Work out the finished part from the listing and answer in its coordinate system (mm). A direction names the side the tool comes from. Coordinates: 2 decimals unless noted, no trailing zeros. Order: outer loops, then holes, each group sorted by start corner. A loop starts at its lowest first (then second) coordinate and runs counter-clockwise, first axis right, second up. Notation, with made-up numbers: (0, 69) -> (55, 69) arc R17 ccw to (55, 75) -> close; hole circle Ø8 at (7, 47.25). An arc over 180 degrees is marked (long way). Answer as CSV lines item,"result". Start each with the question number.
Item 1: Section A-A (y = -0.5) is taken. Write down the section's boundary in (x, z), then the cut area to 3 significant figures.
Item 2: For a pull along X with two mould halves and no side action, classify faces 3 (the face through (3, 4.226, -5)), 4 (the face through (25.591, -5, -5)), 5 (the face through (-22.034, -5, -5)), 6 (the face through (3, 5, -381)) as pulls with the +X half, pulls with the -X half, needs draft (parallel to the pull), parting line crosses it, or undercut.
Item 3: Section B-B (x = 5.5) is taken. Write down the section's boundary in (y, z).
Item 4: Section C-C (z = 318.5) is taken. Write down the section's boundary in (x, y).
Item 5: This flat-tipped pin is pushed along its axis until it touches: pin 1 Ø4.5 at (x, z) = (16.07, 12.7) entering from -Y. Where does it stop, or does it pass through?
Item 6: Straight lines are drawn through the part: L1, parallel to X at y = -15.5, z = -368.3; L2, parallel to Y at x = -14, z = -111; L3, parallel to X at y = -10, z = 224.5. For each, find the intervals that lie inside material, in ascending order.
Item 7: Which of the six approach directions +Z, -Z, +X, -X, +Y, -Y give full straight-line access (tool end or side, diameter ignored) to faces 1 (the face through (28.766, -5, -5)), 2 (the face through (-18.859, -5, -5))?
Autodesk Inventor part; units mm, degrees
ref_plane "YZ Plane" through (0, 0, 0) normal (1, 0, 0) x (0, 1, 0)
ref_plane "XZ Plane" through (0, 0, 0) normal (0, 1, 0) x (-1, 0, 0)
ref_plane "XY Plane" through (0, 0, 0) normal (0, 0, 1) x (1, 0, 0)
sketch "Sketch1" plane through (0, 0, 0) normal (0, 0, 1) x (1, 0, 0)
  line L0 (-22.0343, 7.401) -> (28.7657, 7.401)
  line L1 (28.7657, 7.401) -> (28.7657, -17.999)
  line L2 (28.7657, -17.999) -> (-22.0343, -17.999)
  line L3 (-22.0343, -17.999) -> (-22.0343, 7.401)
  line L4 (-18.8593, 4.226) -> (25.5907, 4.226)
  line L5 (25.5907, 4.226) -> (25.5907, -14.824)
  line L6 (25.5907, -14.824) -> (-18.8593, -14.824)
  line L7 (-18.8593, -14.824) -> (-18.8593, 4.226)
  point P0 (0, 0)
  dimension "d0" = 50.8
  dimension "d1" = 25.4
  dimension "d2" = 3.175
  dimension "d3" = 3.175
  dimension "d4" = 3.175
  dimension "d5" = 3.175
extrude "Extrusion1" add sketch "Sketch1" along normal mid plane 762
sketch "Sketch2" plane through (-22.0343, 7.401, 381) normal (0, 1, 0) x (1, 0, 0)
  line L0 (50.8, 0) -> (0, 0)
  line L1 (0, 762) -> (0, 0)
  point P0 (22.0343, 381)
  point P1 (12.7, 12.7)
  dimension "d8" = 12.7
  dimension "d9" = 12.7
hole "Hole1" at (-9.3343, 7.401, 368.3) direction (0, -1, 0) diameter 4.7625 depth 27.94
sketch "Sketch3" plane through (-22.0343, 7.401, 381) normal (0, 1, 0) x (1, 0, 0)
  line L0 (50.8, 0) -> (0, 0)
  line L1 (50.8, 762) -> (50.8, 0)
  point P0 (22.0343, 381)
  point P1 (38.1, 12.7)
  dimension "d17" = 12.7
  dimension "d18" = 12.7
hole "Hole2" at (16.0657, 7.401, 368.3) direction (0, -1, 0) diameter 4.7625 depth 27.94
sketch "Sketch4" plane through (-22.0343, 7.401, 381) normal (0, 1, 0) x (1, 0, 0)
  line L0 (0, 762) -> (0, 0)
  line L1 (50.8, 0) -> (0, 0)
  point P0 (22.0343, 381)
  point P1 (12.7, 165.1)
  dimension "d26" = 12.7
  dimension "d27" = 165.1
hole "Hole3" at (-9.3343, 7.401, 215.9) direction (0, -1, 0) diameter 4.7625 depth 27.94
sketch "Sketch5" plane through (-22.0343, 7.401, 381) normal (0, 1, 0) x (1, 0, 0)
  line L0 (50.8, 762) -> (50.8, 0)
  line L1 (50.8, 0) -> (0, 0)
  point P0 (22.0343, 381)
  point P1 (38.1, 165.1)
  dimension "d35" = 12.7
  dimension "d36" = 165.1
hole "Hole4" at (16.0657, 7.401, 215.9) direction (0, -1, 0) diameter 4.7625 depth 27.94
sketch "Sketch6" plane through (-22.0343, 7.401, 381) normal (0, 1, 0) x (1, 0, 0)
  line L0 (0, 762) -> (50.8, 762)
  line L1 (0, 762) -> (0, 0)
  point P0 (22.0343, 381)
  point P1 (12.7, 749.3)
  dimension "d44" = 12.7
  dimension "d45" = 12.7
hole "Hole5" at (-9.3343, 7.401, -368.3) direction (0, -1, 0) diameter 4.7625 depth 27.94
sketch "Sketch7" plane through (-22.0343, 7.401, 381) normal (0, 1, 0) x (1, 0, 0)
  line L0 (0, 762) -> (50.8, 762)
  line L1 (50.8, 762) -> (50.8, 0)
  point P0 (22.0343, 381)
  point P1 (38.1, 749.3)
  dimension "d53" = 12.7
  dimension "d54" = 12.7
hole "Hole6" at (16.0657, 7.401, -368.3) direction (0, -1, 0) diameter 4.7625 depth 27.94
sketch "Sketch8" plane through (-22.0343, 7.401, 381) normal (0, 1, 0) x (1, 0, 0)
  line L0 (0, 762) -> (50.8, 762)
  line L1 (0, 762) -> (0, 0)
  point P0 (22.0343, 381)
  point P1 (12.7, 596.9)
  dimension "d62" = 165.1
  dimension "d63" = 12.7
hole "Hole7" at (-9.3343, 7.401, -215.9) direction (0, -1, 0) diameter 4.7625 depth 27.94
sketch "Sketch9" plane through (-22.0343, 7.401, 381) normal (0, 1, 0) x (1, 0, 0)
  line L0 (0, 762) -> (50.8, 762)
  line L1 (50.8, 762) -> (50.8, 0)
  point P0 (22.0343, 381)
  point P1 (38.1, 596.9)
  dimension "d71" = 165.1
  dimension "d72" = 12.7
hole "Hole8" at (16.0657, 7.401, -215.9) direction (0, -1, 0) diameter 4.7625 depth 27.94
sketch "Sketch14" plane through (-22.0343, 7.401, 381) normal (0, 1, 0) x (1, 0, 0)
  line L0 (0, 762) -> (0, 0)
  line L1 (50.8, 0) -> (0, 0)
  point P0 (22.0343, 381)
  point P1 (12.7, 254)
  dimension "d116" = 12.7
  dimension "d117" = 254
hole "Hole13" at (-9.3343, 7.401, 127) direction (0, -1, 0) diameter 4.7625 depth 104.14
sketch "Sketch15" plane through (-22.0343, 7.401, 381) normal (0, 1, 0) x (1, 0, 0)
  line L0 (0, 762) -> (0, 0)
  line L1 (50.8, 0) -> (0, 0)
  point P0 (22.0343, 381)
  point P1 (38.1, 254)
  dimension "d125" = 38.1
  dimension "d126" = 254
hole "Hole14" at (16.0657, 7.401, 127) direction (0, -1, 0) diameter 4.7625 depth 104.14
sketch "Sketch16" plane through (-22.0343, 7.401, 381) normal (0, 1, 0) x (1, 0, 0)
  line L0 (0, 762) -> (0, 0)
  line L1 (50.8, 0) -> (0, 0)
  point P0 (22.0343, 381)
  point P1 (12.7, 228.6)
  dimension "d134" = 12.7
  dimension "d135" = 228.6
hole "Hole15" at (-9.3343, 7.401, 152.4) direction (0, -1, 0) diameter 4.7625 depth 104.14
sketch "Sketch17" plane through (-22.0343, 7.401, 381) normal (0, 1, 0) x (1, 0, 0)
  line L0 (50.8, 0) -> (0, 0)
  line L1 (50.8, 762) -> (50.8, 0)
  point P0 (22.0343, 381)
  point P1 (38.1, 228.6)
  dimension "d143" = 228.6
  dimension "d144" = 12.7
hole "Hole16" at (16.0657, 7.401, 152.4) direction (0, -1, 0) diameter 4.7625 depth 104.14
sketch "Sketch18" plane through (-22.0343, -17.999, 381) normal (0, -1, 0) x (1, 0, 0)
  line L0 (50.8, -762) -> (50.8, 0)
  line L1 (0, 0) -> (50.8, 0)
  point P0 (22.0343, -381)
  point P1 (38.1, -342.9)
  dimension "d152" = 12.7
  dimension "d153" = 342.9
hole "Hole17" at (16.0657, -17.999, 38.1) direction (0, 1, 0) diameter 4.7625 depth 104.14
sketch "Sketch19" plane through (-22.0343, -17.999, 381) normal (0, -1, 0) x (1, 0, 0)
  line L0 (0, 0) -> (0, -762)
  line L1 (0, 0) -> (50.8, 0)
  point P0 (22.0343, -381)
  point P1 (12.7, -342.9)
  dimension "d161" = 12.7
  dimension "d162" = 342.9
hole "Hole18" at (-9.3343, -17.999, 38.1) direction (0, 1, 0) diameter 4.7625 depth 104.14
sketch "Sketch20" plane through (-22.0343, -17.999, 381) normal (0, -1, 0) x (1, 0, 0)
  line L0 (50.8, -762) -> (50.8, 0)
  line L1 (50.8, -762) -> (0, -762)
  point P0 (22.0343, -381)
  point P1 (38.1, -368.3)
  dimension "d170" = 12.7
  dimension "d171" = 393.7
hole "Hole19" at (16.0657, -17.999, 12.7) direction (0, 1, 0) diameter 4.7625 depth 104.14
sketch "Sketch21" plane through (-22.0343, -17.999, 381) normal (0, -1, 0) x (1, 0, 0)
  line L0 (50.8, -762) -> (50.8, 0)
  line L1 (50.8, -762) -> (0, -762)
  point P0 (22.0343, -381)
  point P1 (12.7, -368.3)
  dimension "d179" = 38.1
  dimension "d180" = 393.7
hole "Hole20" at (-9.3343, -17.999, 12.7) direction (0, 1, 0) diameter 4.7625 depth 104.14
equation "\"d4\" = d3"
equation "\"d5\" = d3"
properties part number "HorizontalSupportBar"
Checked values:
1,outline,"(-22.03, -381) -> (-18.86, -381) -> (-18.86, 381) -> (-22.03, 381) -> close; (25.59, -381) -> (28.77, -381) -> (28.77, 381) -> (25.59, 381) -> close"
1,area,"4,840 mm^2"
2,face 3,"undercut"
2,face 4,"undercut"
2,face 5,"pulls with the -X half"
2,face 6,"needs draft"
3,outline,"(-18, -381) -> (-14.82, -381) -> (-14.82, 381) -> (-18, 381) -> close; (4.23, -381) -> (7.4, -381) -> (7.4, 381) -> (4.23, 381) -> close"
4,outline,"(-22.03, -18) -> (28.77, -18) -> (28.77, 7.4) -> (-22.03, 7.4) -> close; hole (-18.86, -14.82) -> (25.59, -14.82) -> (25.59, 4.23) -> (-18.86, 4.23) -> close"
5,pin 1,"passes through"
6,L1,"x = -22.03 to -11.72, -6.95 to 13.68, 18.45 to 28.77"
6,L2,"y = -18 to -14.82, 4.23 to 7.4"
6,L3,"x = -22.03 to -18.86, 25.59 to 28.77"
7,face 1,"+Z, -Z, +X, +Y, -Y"
7,face 2,"+Z, -Z"
